The figure shows three views and two pictorial views of one solid part (mm, origin at its lowest corner). Answer the questions. A direction names the side the tool comes from. Coordinates: 2 decimals unless noted, no trailing zeros. Loops run counter-clockwise (first coordinate to the right, second up) from the corner with the lowest first, then second, coordinate; pieces in that order, holes last. Notation, with made-up numbers: (16, 58) -> (62, 58) arc R14 cw to (62, 83) -> close; hole circle Ø7 at (23, 40.5). An arc over 180 degrees is marked (long way). Answer in a Markdown table with one row per item.
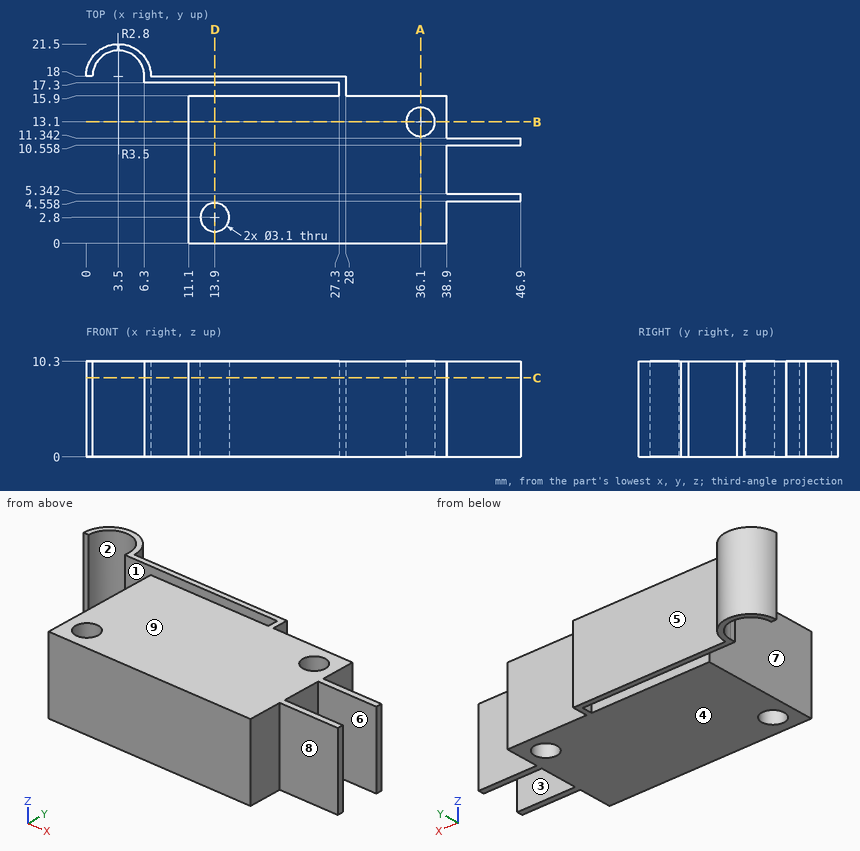
Item 1: A cutting plane is placed at B-B, the plane y = 13.1. Determine the outline of the cut face in (x, z).
Findings below:
| item | result |
|---|---|
| outline | (11.1, 0) -> (34.55, 0) -> (34.55, 10.3) -> (11.1, 10.3) -> close; (37.65, 0) -> (38.9, 0) -> (38.9, 10.3) -> (37.65, 10.3) -> close |
Item 2: A cutting plane is placed at D-D, the plane x = 13.9. Determine the outline of the cut face in (y, z).
Findings below:
| item | result |
|---|---|
| outline | (0, 0) -> (1.25, 0) -> (1.25, 10.3) -> (0, 10.3) -> close; (4.35, 0) -> (15.9, 0) -> (15.9, 10.3) -> (4.35, 10.3) -> close; (17.3, 0) -> (18, 0) -> (18, 10.3) -> (17.3, 10.3) -> close |
Item 3: Flat-ended cylindrical pins translate along their axes: pin 1 Ø2.5 at (x, z) = (44, 5) entering from -Y; pin 2 Ø2 at (y, z) = (12, 4) entering from -X; pin 3 Ø4 at (y, z) = (8.5, 7) entering from +X. Find the tip coordinate at first contact, or state that the pin passes through.
Findings below:
| item | result |
|---|---|
| pin 1 | stops at y = 4.56 |
| pin 2 | stops at x = 11.1 |
| pin 3 | stops at x = 38.9 |
Item 4: A cutting plane is placed at A-A, the plane x = 36.1. Determine the outline of the cut face in (y, z).
Findings below:
| item | result |
|---|---|
| outline | (0, 0) -> (11.55, 0) -> (11.55, 10.3) -> (0, 10.3) -> close; (14.65, 0) -> (15.9, 0) -> (15.9, 10.3) -> (14.65, 10.3) -> close |
Item 5: A cutting plane is placed at C-C, the plane z = 8.5. Determine the outline of the cut face in (x, y).
Findings below:
| item | result |
|---|---|
| outline | (0, 18) -> (0.7, 18) arc R2.8 cw to (6.3, 18) -> (6.3, 17.3) -> (27.3, 17.3) -> (27.3, 15.9) -> (11.1, 15.9) -> (11.1, 0) -> (38.9, 0) -> (38.9, 4.56) -> (46.9, 4.56) -> (46.9, 5.34) -> (38.9, 5.34) -> (38.9, 10.56) -> (46.9, 10.56) -> (46.9, 11.34) -> (38.9, 11.34) -> (38.9, 15.9) -> (28, 15.9) -> (28, 18) -> (7, 18) arc R3.5 ccw to start; hole circle Ø3.1 at (13.9, 2.8); hole circle Ø3.1 at (36.1, 13.1) |
Item 6: Find the intervals of material crossed by probe 1 along Y at (x, z) = (13.9, 6); probe 2 along Y at (x, z) = (36.1, 7.75); probe 3 along Y at (x, z) = (11.5, 1.75), in increasing order.
Findings below:
| item | result |
|---|---|
| probe 1 | y = 0 to 1.25, 4.35 to 15.9, 17.3 to 18 |
| probe 2 | y = 0 to 11.55, 14.65 to 15.9 |
| probe 3 | y = 0 to 15.9, 17.3 to 18 |
Item 7: A tool of negligible diameter and unlimited length cuts with its end or side. For the marked faces 5, 6, 7, 8 and 9, from which of +Z, -Z, +X, -X, +Y, -Y can it reach the whole face along a straight path? Write none if from no direction.
Findings below:
| item | result |
|---|---|
| face 5 | +Z, -Z, +X, +Y |
| face 6 | +Z, -Z, +X |
| face 7 | +Z, -Z, -X, -Y |
| face 8 | +Z, -Z, +X, -Y |
| face 9 | +Z, +X, -X, +Y, -Y |
Item 8: Determine the mould class of the marked faces 1, 2, 3 and 4 for opening direction Y: +Y half, -Y half, draft (parallel to the pull), parting line (faces both ways), or undercut.
Findings below:
| item | result |
|---|---|
| face 1 | undercut |
| face 2 | -Y half |
| face 3 | undercut |
| face 4 | draft |
